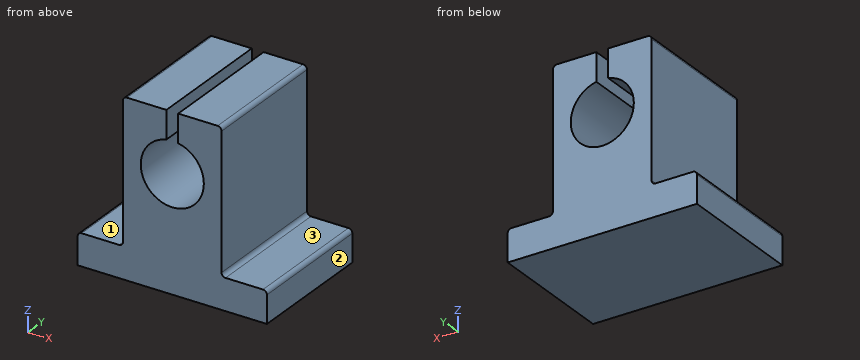
```python
from build123d import *

# Parameters (mm, degrees)
F1_DEPTH = 8
F2_DEPTH = 25


with BuildPart() as f1:
    # F0 (on Front) → F1 (new body, symmetric)
    with BuildSketch(Plane.XZ):
        with BuildLine():
            Line((-24, -12.357661), (-24, -19.357661))
            Line((-24, -19.357661), (24, -19.357661))
            Line((24, -19.357661), (24, -12.357661))
            ThreePointArc((24, -12.357661), (23.707107, -11.650554), (23, -11.357661))
            Line((23, -11.357661), (13.5, -11.357661))
            ThreePointArc((13.5, -11.357661), (12.792893, -11.064767), (12.5, -10.357661))
            Line((12.5, -10.357661), (12.5, 23.642339))
            ThreePointArc((12.5, 23.642339), (12.207107, 24.349446), (11.5, 24.642339))
            Line((11.5, 24.642339), (1.5, 24.642339))
            Line((1.5, 24.642339), (1.5, 17.500456))
            ThreePointArc((1.5, 17.500456), (0, 1.642339), (-1.5, 17.500456))
            Line((-1.5, 17.500456), (-1.5, 24.642339))
            Line((-1.5, 24.642339), (-11.5, 24.642339))
            ThreePointArc((-11.5, 24.642339), (-12.207107, 24.349446), (-12.5, 23.642339))
            Line((-12.5, 23.642339), (-12.5, -10.357661))
            ThreePointArc((-12.5, -10.357661), (-12.792893, -11.064767), (-13.5, -11.357661))
            Line((-13.5, -11.357661), (-23, -11.357661))
            ThreePointArc((-23, -11.357661), (-23.707107, -11.650554), (-24, -12.357661))
        make_face()
    extrude(amount=F1_DEPTH, both=True)

    # F0 (on Front) → F2 (join)
    with BuildSketch(Plane.XZ):
        with BuildLine():
            Line((-24, -12.357661), (-24, -19.357661))
            Line((-24, -19.357661), (24, -19.357661))
            Line((24, -19.357661), (24, -12.357661))
            ThreePointArc((24, -12.357661), (23.707107, -11.650554), (23, -11.357661))
            Line((23, -11.357661), (13.5, -11.357661))
            ThreePointArc((13.5, -11.357661), (12.792893, -11.064767), (12.5, -10.357661))
            Line((12.5, -10.357661), (12.5, 23.642339))
            ThreePointArc((12.5, 23.642339), (12.207107, 24.349446), (11.5, 24.642339))
            Line((11.5, 24.642339), (1.5, 24.642339))
            Line((1.5, 24.642339), (1.5, 17.500456))
            ThreePointArc((1.5, 17.500456), (0, 1.642339), (-1.5, 17.500456))
            Line((-1.5, 17.500456), (-1.5, 24.642339))
            Line((-1.5, 24.642339), (-11.5, 24.642339))
            ThreePointArc((-11.5, 24.642339), (-12.207107, 24.349446), (-12.5, 23.642339))
            Line((-12.5, 23.642339), (-12.5, -10.357661))
            ThreePointArc((-12.5, -10.357661), (-12.792893, -11.064767), (-13.5, -11.357661))
            Line((-13.5, -11.357661), (-23, -11.357661))
            ThreePointArc((-23, -11.357661), (-23.707107, -11.650554), (-24, -12.357661))
        make_face()
    extrude(amount=F2_DEPTH)


solid = f1.part
```
Source: CAD feature listing. Evaluate the final solid. Frame: model axes, mm. Face numbers are marked on the shaded views. A direction names the side the tool comes from. Coordinates: 2 decimals unless noted, no trailing zeros. Loops run counter-clockwise (first coordinate to the right, second up) from the corner with the lowest first, then second, coordinate; pieces in that order, holes last. Notation, with made-up numbers: M 87.25,53.5 L 136.25,53.5 A21 ccw 136.25,80.5 Z; hole C 29,64 d4. An arc over 180 degrees is marked long. Put each result on its own line as item: value. Start each with the question number.
1) Cut plane D-D on z = -5.5. Return the cut outline in (x, y).
2) Contact query for flat-ended pins moving along their axis: pin 1 Ø10 at (y, z) = (-7, -1.5) entering from -X; pin 2 Ø4 at (y, z) = (1, -8) entering from +X; pin 3 Ø5 at (x, y) = (16, -15) entering from +Z. Output: stop coordinate, or through.
3) Cut plane A-A on x = -3. Return the cut outline in (y, z).
4) Reachability of the marked faces 1, 2 and 3 from +Z, -Z, +X, -X, +Y, -Y: full face, straight path, thin tool, end or side. Return the list, or none.
5) Cut plane B-B on y = -17. Return the cut outline in (x, z).
6) Ray query, L1, parallel to X at y = -4.5, z = 22.5; L2, parallel to Z at x = 0, y = -10.5; L3, parallel to X at y = -6, z = 5.5. Return the intervals inside material, ascending. Write a range as from..to.
7) Cut plane C-C on x = -16. Return the cut outline in (y, z).
The answers:
1. outline: M -12.5,-25 L 12.5,-25 L 12.5,8 L -12.5,8 Z
2. pin 1: stops at x = -12.5
2. pin 2: stops at x = 12.5
2. pin 3: stops at z = -11.36
3. outline: M -25,-19.36 L 8,-19.36 L 8,2.23 L -25,2.23 Z; M -25,17.06 L 8,17.06 L 8,24.64 L -25,24.64 Z
4. face 1: +Z, -X, +Y, -Y
4. face 2: +Z, -Z, +X, +Y, -Y
4. face 3: +Z, +X, +Y, -Y
5. outline: M -24,-19.36 L 24,-19.36 L 24,-12.36 A1 ccw 23,-11.36 L 13.5,-11.36 A1 cw 12.5,-10.36 L 12.5,23.64 A1 ccw 11.5,24.64 L 1.5,24.64 L 1.5,17.5 A8 cw long -1.5,17.5 L -1.5,24.64 L -11.5,24.64 A1 ccw -12.5,23.64 L -12.5,-10.36 A1 cw -13.5,-11.36 L -23,-11.36 A1 ccw -24,-12.36 Z
6. L1: x = -12.5..-1.5, 1.5..12.5
6. L2: z = -19.36..1.64
6. L3: x = -12.5..-6.84, 6.84..12.5
7. outline: M -25,-19.36 L 8,-19.36 L 8,-11.36 L -25,-11.36 Z
